Verification items for the finished model (mm, model axes). Give positions to 0.01 mm unless a question says otherwise; leave off trailing zeros. Order: outer loops, then holes, each group sorted by start corner. A loop starts at its lowest first (then second) coordinate and runs counter-clockwise, first axis right, second up. Notation, with made-up numbers: M 79.5,70 L 97.5,70 A17 cw 97.5,80 Z; hole C 39.5,-10 d1. An arc over 180 degrees is marked long. Answer as a JSON object with one key per item and string values.
```python
from build123d import *

# Parameters (mm, degrees)
F0_R          = 76.2
F1_DEPTH      = 50.8
F1_DEPTH_BACK = 50.8
F2_R          = 25.4
F3_DEPTH      = 101.601
F4_SIZE       = 12.7
F5_R          = 10.297763
F6_DEPTH      = 152.4


with BuildPart() as f1:
    # F0 (on Front) → F1 (new body, two sides)
    with BuildSketch(Plane.XZ) as f1_sk:
        Circle(F0_R)
    extrude(amount=F1_DEPTH)
    extrude(f1_sk.sketch, amount=-F1_DEPTH_BACK)

    # F2 (on face) → F3 (cut, through all)
    with BuildSketch(Plane.XZ.offset(50.8)):
        Circle(F2_R)
    extrude(amount=-F3_DEPTH, mode=Mode.SUBTRACT)

    # F4
    f4_edges = [f1.edges().sort_by_distance(p)[0] for p in [
        (-76.2, -50.8, 0),
        (-76.2, 50.8, 0),
    ]]
    chamfer(f4_edges, length=F4_SIZE)

    # F5 (on Right) → F6 (cut, symmetric)
    with BuildSketch(Plane.YZ):
        Circle(F5_R)
    extrude(amount=F6_DEPTH, both=True, mode=Mode.SUBTRACT)


solid = f1.part
```
Q1. Section check B-B on x = 0. Record the cut outline in (y, z), then the cut area to 4 significant figures.
Resolved:
{"outline": "M -50.8,-63.5 L -38.1,-76.2 L 38.1,-76.2 L 50.8,-63.5 L 50.8,-25.4 L -50.8,-25.4 Z; M -50.8,25.4 L 50.8,25.4 L 50.8,63.5 L 38.1,76.2 L -38.1,76.2 L -50.8,63.5 Z", "area": "10,000 mm²"}
Q2. Release check for a two-part mould opening along Z. For faces 1 (the face through (72.68, -0.53, 22.89)), 2 (the face through (27, 50.8, 1)), 3 (the face through (50.08, -8.17, -6.27)) record: +Z half, -Z half, draft (parallel to the pull), parting line (faces both ways), or undercut.
Resolved:
{"face 1": "parting line", "face 2": "draft", "face 3": "undercut"}
Q3. Material ranges on L1, parallel to Y at x = 52, z = 0; L2, parallel to Z at x = 0, y = 6, recorded low to high.
Resolved:
{"L1": "y = -50.8 to -10.3, 10.3 to 50.8", "L2": "z = -76.2 to -25.4, 25.4 to 76.2"}
Q4. Section check D-D on y = 21.5. Record the cut outline in (x, z).
Resolved:
{"outline": "C 0,0 d152.4; hole C 0,0 d50.8"}
Q5. Section check C-C on y = 0. Record the cut outline in (x, z), then the cut area to 3 significant figures.
Resolved:
{"outline": "M -75.5,-10.3 A76.2 ccw 75.5,-10.3 L 23.22,-10.3 A25.4 cw -23.22,-10.3 Z; M -75.5,10.3 L -23.22,10.3 A25.4 cw 23.22,10.3 L 75.5,10.3 A76.2 ccw Z", "area": "14,100 mm²"}
Q6. Gauge pin test, flat ends, axial feed: pin 1 Ø6 at (x, y) = (-53, 34) entering from -Z; pin 2 Ø3 at (x, z) = (36.5, 54) entering from +Y; pin 3 Ø4 at (x, y) = (-55, -25) entering from +Z; pin 4 Ø12.5 at (y, z) = (0, 0) entering from +X. Record the tip position at first contact, or that the pin passes through.
Resolved:
{"pin 1": "stops at z = -57.5", "pin 2": "stops at y = 50.62", "pin 3": "stops at z = 54.75", "pin 4": "passes through"}
Q7. Section check A-A on z = 0. Record the cut outline in (x, y), then the cut area to 3 significant figures.
Resolved:
{"outline": "M -76.2,-38.1 L -63.5,-50.8 L -25.4,-50.8 L -25.4,-10.3 L -76.2,-10.3 Z; M -76.2,10.3 L -25.4,10.3 L -25.4,50.8 L -63.5,50.8 L -76.2,38.1 Z; M 25.4,-50.8 L 63.5,-50.8 L 76.2,-38.1 L 76.2,-10.3 L 25.4,-10.3 Z; M 25.4,10.3 L 76.2,10.3 L 76.2,38.1 L 63.5,50.8 L 25.4,50.8 Z", "area": "7,910 mm²"}
